from build123d import *

# Parameters (mm, degrees)
BOSS_EXTRUDE1_DEPTH = 7
SKETCH2_R           = 2.7
CUT_EXTRUDE1_DEPTH  = 4
SKETCH4_R           = 2
CUT_EXTRUDE2_DEPTH  = 10


with BuildPart() as part:
    # Sketch1 → Boss-Extrude1 (new body)
    with BuildSketch(Plane.XY):
        with BuildLine():
            Line((-20, 0), (-20, 7))
            Line((-20, 7), (-23, 7))
            Line((-23, 7), (-23, 0))
            ThreePointArc((-23, 0), (-16.263455967, -16.263455967), (0, -23))
            Line((0, -23), (7, -23))
            Line((7, -23), (7, -20))
            Line((7, -20), (0, -20))
            ThreePointArc((0, -20), (-14.142135624, -14.142135624), (-20, 0))
        make_face()
    extrude(amount=BOSS_EXTRUDE1_DEPTH)

    # Sketch2 → Cut-Extrude1 (cut, through all)
    with BuildSketch(Plane(origin=(-20, 0, 0), x_dir=(0, 0, -1), z_dir=(1, 0, 0))):
        with Locations((-3.5, 3.5)):
            Circle(SKETCH2_R)
    extrude(amount=-CUT_EXTRUDE1_DEPTH, mode=Mode.SUBTRACT)

    # Sketch4 → Cut-Extrude2 (cut)
    with BuildSketch(Plane(origin=(0, -20, 0), x_dir=(1, 0, 0), z_dir=(0, 1, 0))):
        with Locations((3.5, -3.5)):
            Circle(SKETCH4_R)
    extrude(amount=-CUT_EXTRUDE2_DEPTH, mode=Mode.SUBTRACT)


solid = part.part
Model file for the job. Use its own axes, mm. A direction names the side the tool comes from. Coordinates: 2 decimals unless noted, no trailing zeros. Loops run counter-clockwise (first coordinate to the right, second up) from the corner with the lowest first, then second, coordinate; pieces in that order, holes last. Notation, with made-up numbers: (50, -29) -> (58, -29) arc R25 cw to (58, 4) -> close; hole circle Ø3 at (-6, 42.25). An arc over 180 degrees is marked (long way). Use one line per item in the form item = value. Start each with the question number.
(1) Pull direction Y, two halves, no side cores. Call faces 3 (the flat face through (5.1, -20, 5)), 4 (the cylindrical face through (-21.479, 1.105, 2.254)), 5 (the flat face through (-15, -15, 0)): pulls with the +Y half, pulls with the -Y half, needs draft (parallel to the pull), parting line crosses it, or undercut.
(2) Tool access for faces 1 (the flat face through (-20, 1, 5)), 2 (the flat face through (-23, 2, 1)): list every direction of +Z, -Z, +X, -X, +Y, -Y with a clear straight run to the whole face (end or side of a thin tool).
(3) Cut at A-A on y = 3.5. Give the cut face in (x, z).
(4) Cut at D-D on y = -13. Give the cut face in (x, z), and give its area (3 significant figures).
(5) Flat gauge pins, fed straight in: pin 1 (1.5 mm diameter, centred on y = -15, z = 3, fed in from -X); pin 2 (10 mm diameter, centred on x = -3, y = -10, fed in from +Z); pin 3 (2 mm diameter, centred on x = -16.5, y = -10.5, fed in from +Z); pin 4 (3 mm diameter, centred on x = 1, z = 5.5, fed in from +Y). Where does each tip first touch, or does it go through?
(6) Probe probe 1 along Z at (x, y) = (3.5, -22.1); probe 2 along X at (y, z) = (-21.2, 3.5); probe 3 along Y at (x, z) = (-20.7, 3.5). List the from-to ranges inside material, lowest first. Write a range as from..to.
(7) Cut at C-C on z = 3.5. Give the cut face in (x, y), and give its area (3 significant figures).
(8) Cut at B-B on x = 3.5. Give the cut face in (y, z), and give its area (3 significant figures).
Values:
q1.face_3 = pulls with the +Y half
q1.face_4 = undercut
q1.face_5 = needs draft
q2.face_1 = +Z, -Z, +X, +Y
q2.face_2 = +Z, -Z, -X, +Y, -Y
q3.outline = (-23, 0) -> (-20, 0) -> (-20, 0.8) -> (-23, 0.8) -> close; (-23, 6.2) -> (-20, 6.2) -> (-20, 7) -> (-23, 7) -> close
q4.outline = (-18.97, 0) -> (-15.2, 0) -> (-15.2, 7) -> (-18.97, 7) -> close
q4.area = 26.4 mm2
q5.pin_1 = -18.05
q5.pin_2 = through
q5.pin_3 = 7
q5.pin_4 = -19.99
q6.probe_1 = 0..1.5, 5.5..7
q6.probe_2 = -8.92..1.5, 5.5..7
q6.probe_3 = -10.03..0.8, 6.2..7
q7.outline = (-23, 0) arc R23 ccw to (0, -23) -> (1.5, -23) -> (1.5, -20) -> (0, -20) arc R20 cw to (-20, 0) -> (-20, 0.8) -> (-23, 0.8) -> close; (-23, 6.2) -> (-20, 6.2) -> (-20, 7) -> (-23, 7) -> close; (5.5, -23) -> (7, -23) -> (7, -20) -> (5.5, -20) -> close
q7.area = 115 mm2
q8.outline = (-23, 0) -> (-20, 0) -> (-20, 1.5) -> (-23, 1.5) -> close; (-23, 5.5) -> (-20, 5.5) -> (-20, 7) -> (-23, 7) -> close
q8.area = 9.00 mm2
